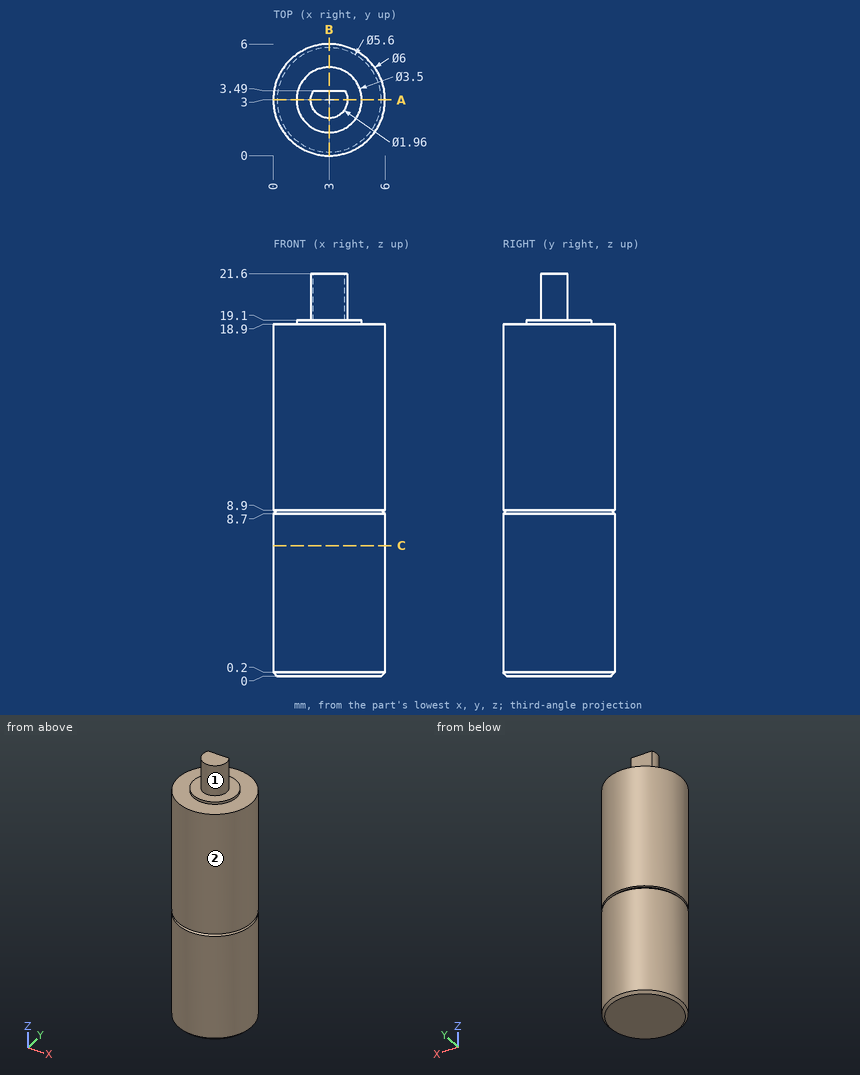
Answer from the drawing. Dimensions are ordinates in mm from the lowest x, y and z of the part. A direction names the side the tool comes from. Round coordinates to 2 decimals unless told otherwise and drop trailing zeros. Write each loop counter-clockwise with the first axis right and the second up, starting at its lowest first coordinate (ties: lowest second). Pieces come first, ordered by that corner, then holes. Notation, with made-up numbers: (22.5, -34.75) -> (49.5, -34.75) arc R17 ccw to (49.5, -19.75) -> close; hole circle Ø10 at (-22.5, 1.25). An arc over 180 degrees is marked (long way). Write each question's results on one line, items separated by ' | '.
1) Flat-ended cylindrical pins translate along their axes: pin 1 (1 mm diameter, centred on x = 5.5, z = 17.5, fed in from -Y); pin 2 (1 mm diameter, centred on x = 0.5, z = 11.5, fed in from +Y); pin 3 (0.8 mm diameter, centred on x = 3, z = 20, fed in from +Y). Find the tip coordinate at first contact, or state that the pin passes through.
Findings:
pin 1: stops at y = 0.76 | pin 2: stops at y = 5.24 | pin 3: stops at y = 3.49
2) Consider line 1 along Z through (x, y) = (1.95, 4.85); line 2 along Z through (x, y) = (2.25, 4.25); line 3 along X through (y, z) = (1.5, 14.75). Determine where each line is inside the solid, lowest interval first. Write a range as [from, to].
Findings:
line 1: z = [0, 18.9] | line 2: z = [0, 19.1] | line 3: x = [0.4, 5.6]
3) Which of the six approach directions +Z, -Z, +X, -X, +Y, -Y give full straight-line access (tool end or side, diameter ignored) to the marked faces 1 and 2?
Findings:
face 1: +Z | face 2: +Z, -Z
4) The part is cut by section B-B (x = 3). Write down the section's boundary in (y, z).
Findings:
outline: (0, 0.2) -> (0.2, 0) -> (5.8, 0) -> (6, 0.2) -> (6, 8.7) -> (5.8, 8.9) -> (6, 8.9) -> (6, 18.9) -> (4.75, 18.9) -> (4.75, 19.1) -> (3.49, 19.1) -> (3.49, 21.6) -> (2.02, 21.6) -> (2.02, 19.1) -> (1.25, 19.1) -> (1.25, 18.9) -> (0, 18.9) -> (0, 8.9) -> (0.2, 8.9) -> (0, 8.7) -> close
5) The part is cut by section C-C (z = 7). Write down the section's boundary in (x, y), and give its area (3 significant figures).
Findings:
outline: circle Ø6 at (3, 3) | area: 28.3 mm²
6) The part is cut by section A-A (y = 3). Write down the section's boundary in (x, z).
Findings:
outline: (0, 0.2) -> (0.2, 0) -> (5.8, 0) -> (6, 0.2) -> (6, 8.7) -> (5.8, 8.9) -> (6, 8.9) -> (6, 18.9) -> (4.75, 18.9) -> (4.75, 19.1) -> (3.98, 19.1) -> (3.98, 21.6) -> (2.02, 21.6) -> (2.02, 19.1) -> (1.25, 19.1) -> (1.25, 18.9) -> (0, 18.9) -> (0, 8.9) -> (0.2, 8.9) -> (0, 8.7) -> close
